Check sheet for the modelled part. Datum: model origin and axes. Units: mm. Round coordinates to 2 decimals unless told otherwise and drop trailing zeros. Order: outer loops, then holes, each group sorted by start corner. A loop starts at its lowest first (then second) coordinate and runs counter-clockwise, first axis right, second up.
Q1. Scan lines: probe 1 along X at (y, z) = (3, 0) (3 decimals); probe 2 along X at (y, z) = (3.75, -15.24); probe 3 along X at (y, z) = (3.75, 15.5). Record each from-to range of solid material in increasing order.
Q2. Cross-section at C-C on y = 2. Give the number of separate pieces and of enclosed holes in the cut face, then the cut area to 3 significant figures.
Q3. Depth check by flat-ended pin: P1, Ø2, axis at x = -34.29, z = -15.24, coming from the +Y side. Enter the tip coordinate at first touch or a pass-through.
Q4. Cross-section at D-D on z = 7.5. Record the cut outline in (x, y), then the cut area to 3 significant figures.
Q5. Cross-section at A-A on z = 0. Record the cut outline in (x, y) (3 decimals).
Q6. Cross-section at B-B on x = 97.79. Record the cut outline in (y, z) (3 decimals), then the cut area to 3 significant figures.
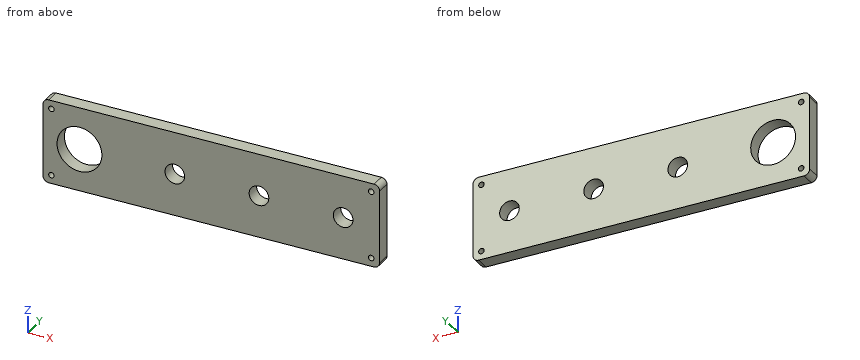
from build123d import *

# Parameters (mm, degrees)
SKETCH1_R             = 4.445
SKETCH1_R_2           = 10.16
BOSS_EXTRUDE1_DEPTH   = 6.35
M3X0_5_TAPPED_HOLE1_D = 2.5


with BuildPart() as part:
    # Sketch1 → Boss-Extrude1 (new body)
    with BuildSketch(Plane.XZ):
        with BuildLine():
            Line((-35.56, -19.05), (111.76, -19.05))
            ThreePointArc((111.76, -19.05), (113.556051224, -18.306051224), (114.3, -16.51))
            Line((114.3, -16.51), (114.3, 16.51))
            ThreePointArc((114.3, 16.51), (113.556051224, 18.306051224), (111.76, 19.05))
            Line((111.76, 19.05), (-35.56, 19.05))
            ThreePointArc((-35.56, 19.05), (-37.356051224, 18.306051224), (-38.1, 16.51))
            Line((-38.1, 16.51), (-38.1, -16.51))
            ThreePointArc((-38.1, -16.51), (-37.356051224, -18.306051224), (-35.56, -19.05))
        make_face()
        with Locations(Location((59.69, 0, 0), (0, 0, 270))):
            Circle(SKETCH1_R, mode=Mode.SUBTRACT)
        with Locations(Location((97.79, 0, 0), (0, 0, 270))):
            Circle(SKETCH1_R, mode=Mode.SUBTRACT)
        with Locations(Location((21.59, 0, 0), (0, 0, 90))):
            Circle(SKETCH1_R, mode=Mode.SUBTRACT)
        with Locations(Location((-21.59, 0, 0), (0, 0, 90))):
            Circle(SKETCH1_R_2, mode=Mode.SUBTRACT)
    extrude(amount=-BOSS_EXTRUDE1_DEPTH)

    # M3x0.5 Tapped Hole1 (through all)
    with Locations(Plane(origin=(0, 6.35, 0), x_dir=(1, 0, 0), z_dir=(0, 1, 0))):
        with Locations((-34.29, 15.24), (110.49, 15.24), (110.49, -15.24), (-34.29, -15.24)):
            Hole(M3X0_5_TAPPED_HOLE1_D / 2)


solid = part.part
Results found:
1. probe 1: x = -38.1 to -31.75, -11.43 to 17.145, 26.035 to 55.245, 64.135 to 93.345, 102.235 to 114.3
1. probe 2: x = -38.1 to -35.54, -33.04 to 109.24, 111.74 to 114.3
1. probe 3: x = -38.1 to -35.51, -33.07 to 109.27, 111.71 to 114.3
2. separate pieces: 1
2. enclosed holes: 8
2. area: 5,270 mm2
3. P1: passes through
4. outline: (-38.1, 0) - (-28.44, 0) - (-28.44, 6.35) - (-38.1, 6.35) - close; (-14.74, 0) - (114.3, 0) - (114.3, 6.35) - (-14.74, 6.35) - close
4. area: 881 mm2
5. outline: (-38.1, 0) - (-31.75, 0) - (-31.75, 6.35) - (-38.1, 6.35) - close; (-11.43, 0) - (17.145, 0) - (17.145, 6.35) - (-11.43, 6.35) - close; (26.035, 0) - (55.245, 0) - (55.245, 6.35) - (26.035, 6.35) - close; (64.135, 0) - (93.345, 0) - (93.345, 6.35) - (64.135, 6.35) - close; (102.235, 0) - (114.3, 0) - (114.3, 6.35) - (102.235, 6.35) - close
6. outline: (0, -19.05) - (6.35, -19.05) - (6.35, -4.445) - (0, -4.445) - close; (0, 4.445) - (6.35, 4.445) - (6.35, 19.05) - (0, 19.05) - close
6. area: 185 mm2
